```python
from build123d import *

# Parameters (mm, degrees)
EXTRUDE_1_DEPTH     = 22
SKETCH_2_W          = 32.061557032
SKETCH_2_H          = 43.504749412
CUT_EXTRUDE_1_DEPTH = 16
SKETCH_3_W          = 6
SKETCH_3_H          = 10.337049688
CUT_EXTRUDE_2_DEPTH = 30
SKETCH_9_R          = 2.5
CUT_EXTRUDE_4_DEPTH = 37.263066611
HOLE_WIZARD_M4_1_D  = 3.3
CHAMFER_1_SIZE      = 12
CHAMFER_1_SIZE_2    = 5
FILLET_2_R          = 3
FILLET_3_R          = 3
FILLET_4_R          = 1


with BuildPart() as part:
    # 草圖1 → 填料-伸長1 (new body)
    with BuildSketch(Plane.XY):
        Polygon((0, 0), (3, 0), (3, 9.7), (9, 9.7), (9, 0), (12, 0), (12, 27.4), (9, 27.4), (9, 21.7), (3, 21.7), (3, 27.4), (0, 27.4), align=None)
    extrude(amount=EXTRUDE_1_DEPTH)

    # 草圖2 → 除料-伸長1 (cut)
    with BuildSketch(Plane(origin=(0, 0, 0), x_dir=(0, 0, -1), z_dir=(1, 0, 0))):
        with Locations((-6.749670429, 14.217142955)):
            Rectangle(SKETCH_2_W, SKETCH_2_H)
        with BuildLine():
            Line((-20.5, 9.7), (-10, 9.7))
            ThreePointArc((-10, 9.7), (-9.292893219, 9.407106781), (-9, 8.7))
            Line((-9, 8.7), (-9, 4.5))
            ThreePointArc((-9, 4.5), (-3.620541034, 0.086775337), (-0.343754699, 6.225))
            ThreePointArc((-0.343754699, 6.225), (-1.833358396, 13.7), (-0.343754699, 21.175))
            ThreePointArc((-0.343754699, 21.175), (-3.620541034, 27.313224663), (-9, 22.9))
            Line((-9, 22.9), (-9, 21.7))
            Line((-9, 21.7), (-20.5, 21.7))
            Line((-20.5, 21.7), (-20.5, 9.7))
        make_face(mode=Mode.SUBTRACT)
    extrude(amount=CUT_EXTRUDE_1_DEPTH, mode=Mode.SUBTRACT)

    # 草圖3 → 除料-伸長2 (cut)
    with BuildSketch(Plane(origin=(0, 0, 0), x_dir=(1, 0, 0), z_dir=(0, 1, 0))):
        with Locations((6, -5.331475156)):
            Rectangle(SKETCH_3_W, SKETCH_3_H)
    extrude(amount=CUT_EXTRUDE_2_DEPTH, mode=Mode.SUBTRACT)

    # 草圖9 → 除料-伸長4 (cut, through all)
    with BuildSketch(Plane(origin=(12, 0, 0), x_dir=(0, 0, -1), z_dir=(1, 0, 0))):
        with Locations((-4.5, 4.5)):
            Circle(SKETCH_9_R)
        with Locations((-4.5, 22.9)):
            Circle(SKETCH_9_R)
    extrude(amount=-CUT_EXTRUDE_4_DEPTH, mode=Mode.SUBTRACT)

    # M4 螺紋孔1 (through all)
    with Locations(Plane(origin=(12, 0, 0), x_dir=(0, 0, -1), z_dir=(1, 0, 0))):
        with Locations((-17.5, 14.2)):
            Hole(HOLE_WIZARD_M4_1_D / 2)

    # 導角1
    # the kernel refuses this chamfer: 12, 5 mm, written as the material it takes off along each edge
    with BuildSketch(Plane(origin=(43.111115995, 21.7, 20.5), x_dir=(0, 0.014835162506254055, -0.9998899529215268), z_dir=(-1, 0, 0))) as chamfer_1_piece_1_section:
        Polygon((CHAMFER_1_SIZE * 0.999889952922, CHAMFER_1_SIZE * 0.0148351625063), (-CHAMFER_1_SIZE_2 * 0.0148351625063, CHAMFER_1_SIZE_2 * 0.999889952922), (0, 0), align=None)
    chamfer_1_piece_1 = extrude(amount=74.22223199, mode=Mode.PRIVATE)
    chamfer_1_piece_1 = split(chamfer_1_piece_1, bisect_by=Plane(origin=(10.5, 21.408333333, 9), z_dir=(0, 0, 1)), keep=Keep.TOP, mode=Mode.PRIVATE)
    add(chamfer_1_piece_1, mode=Mode.SUBTRACT)

    # 圓角2
    fillet_2_edges = [part.edges().sort_by_distance(p)[0] for p in [
        (6, 9.7, 20.5),
    ]]
    fillet(fillet_2_edges, radius=FILLET_2_R)

    # 圓角3
    fillet_3_edges = [part.edges().sort_by_distance(p)[0] for p in [
        (6, 16.7, 20.5),
    ]]
    fillet(fillet_3_edges, radius=FILLET_3_R)

    # 圓角4
    fillet_4_edges = [part.edges().sort_by_distance(p)[0] for p in [
        (1.5, 21.491666667, 9),
        (10.5, 21.491666667, 9),
    ]]
    fillet(fillet_4_edges, radius=FILLET_4_R)


solid = part.part
```
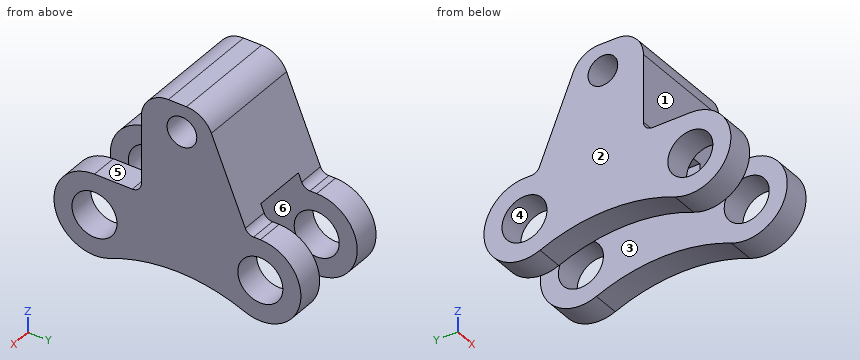
Part model, mm, in its own coordinate system. Face numbers are marked on the shaded views. A direction names the side the tool comes from. Coordinates: 2 decimals unless noted, no trailing zeros. Loops run counter-clockwise (first coordinate to the right, second up) from the corner with the lowest first, then second, coordinate; pieces in that order, holes last. Notation, with made-up numbers: (39.25, 10) - (81.25, 10) arc R21 cw to (81.25, 29) - close; hole circle Ø8 at (71.25, -34). An arc over 180 degrees is marked (long way). Write item = value, one per line. Start each with the question number.
Item 1: Wall check: L1, parallel to Y at x = 9.7, z = 4.5; L2, parallel to X at y = 13.75, z = 3.25; L3, parallel to Y at x = 11.25, z = 3.75. Give the ranges that are in metal, low to high. Write a range as from..to.
Item 2: Cut at B-B, the plane z = 4.5. Give the cut face in (x, y), and give its area (3 significant figures).
Item 3: Mould opens along Z. For the marked faces 4, 5 and 6 say: released by +Z, released by -Z, zero draft, split by the parting line, or undercut.
Item 4: Cut at D-D, the plane x = 6.5. Give the cut face in (y, z).
Item 5: Flat gauge pins, fed straight in: pin 1 Ø5 at (x, y) = (9, 24.5) entering from -Z; pin 2 Ø2.5 at (x, y) = (10, 6) entering from +Z; pin 3 Ø2 at (x, z) = (4, 12.5) entering from -Y; pin 4 Ø1.8 at (x, y) = (7, 17) entering from -Z. Where does each tip first touch, or does it go through?
Item 6: 3-axis set-ups, long thin cutter, end or side, ignore diameter. For the marked faces 1, 2 and 3: which of +Z, -Z, +X, -X, +Y, -Y reach the whole face in a straight line?
Item 7: Cut at A-A, the plane x = 9.75. Give the cut face in (y, z) (3 decimals).
Item 8: Cut at C-C, the plane y = 2.75. Give the cut face in (x, z).
The answers:
q1.L1 = 0..2, 7..20.4, 25.4..27.4
q1.L2 = 0..3, 9..12
q1.L3 = 0.06..2.12, 6.88..20.52, 25.28..27.34
q2.outline = (0, 0) - (3, 0) - (3, 2) - (0, 2) - close; (0, 7) - (3, 7) - (3, 20.4) - (0, 20.4) - close; (0, 25.4) - (3, 25.4) - (3, 27.4) - (0, 27.4) - close; (9, 0) - (12, 0) - (12, 2) - (9, 2) - close; (9, 7) - (12, 7) - (12, 20.4) - (9, 20.4) - close; (9, 25.4) - (12, 25.4) - (12, 27.4) - (9, 27.4) - close
q2.area = 104 mm2
q3.face_4 = undercut
q3.face_5 = released by +Z
q3.face_6 = zero draft
q4.outline = (9.7, 10.5) - (20.87, 10.5) - (17.47, 18.65) arc R3 ccw to (14.7, 20.5) - (12.7, 20.5) arc R3 ccw to (9.7, 17.5) - close; hole circle Ø3.3 at (14.2, 17.5)
q5.pin_1 = 0
q5.pin_2 = 9
q5.pin_3 = 9.7
q5.pin_4 = 10.5
q6.face_1 = +Z, +X, -X, -Y
q6.face_2 = +Z, -Z, -X, +Y, -Y
q6.face_3 = -Z, +Y, -Y
q7.outline = (4.5, 9) arc R4.5 ccw (long way) to (6.225, 0.344) arc R19.5 cw to (21.175, 0.344) arc R4.5 ccw (long way) to (22.9, 9) - (22.158, 9) arc R1 cw to (21.235, 9.615) - (17.469, 18.654) arc R3 ccw to (14.7, 20.5) - (12.7, 20.5) arc R3 ccw to (9.7, 17.5) - (9.7, 10) arc R1 cw to (8.7, 9) - close; hole circle Ø5 at (4.5, 4.5); hole circle Ø3.3 at (14.2, 17.5); hole circle Ø5 at (22.9, 4.5)
q8.outline = (0, 0.35) - (3, 0.35) - (3, 2.71) - (0, 2.71) - close; (0, 6.29) - (3, 6.29) - (3, 8.65) - (0, 8.65) - close; (9, 0.35) - (12, 0.35) - (12, 2.71) - (9, 2.71) - close; (9, 6.29) - (12, 6.29) - (12, 8.65) - (9, 8.65) - close
